from build123d import *

# Parameters (mm, degrees)
F0_W     = 254
F0_H     = 127
F1_DEPTH = 76.2
F2_W     = 25.4
F2_H     = 76.2
F3_DEPTH = 255.778
F5_D     = 38.1
F6_D     = 38.1
F7_D     = 38.1


with BuildPart() as f1:
    # F0 (on Front) → F1 (new body)
    with BuildSketch(Plane.XZ):
        with Locations((-2.316557, -18.004625)):
            Rectangle(F0_W, F0_H)
    extrude(amount=F1_DEPTH)

    # F2 (on face) → F3 (cut)
    with BuildSketch(Plane.YZ.offset(124.683443)):
        with Locations((-63.5, 7.395375)):
            Rectangle(F2_W, F2_H)
    extrude(amount=-F3_DEPTH, mode=Mode.SUBTRACT)

    # F5 (through all)
    with Locations(Plane.XZ.offset(50.8)):
        with Locations((-103.916557, 20.095375)):
            Hole(F5_D / 2)

    # F6 (through all)
    with Locations(Plane.XZ.offset(50.8)):
        with Locations((-53.116557, 20.095375)):
            Hole(F6_D / 2)

    # F7 (through all)
    with Locations(Plane.XZ.offset(50.8)):
        with Locations((-2.316557, 20.095375), (48.483443, 20.095375), (99.283443, 20.095375)):
            Hole(F7_D / 2)


solid = f1.part
Read the model definition and answer for the solid it produces. Units are mm, in the model's axes. A direction names the side the tool comes from. Coordinates: 2 decimals unless noted, no trailing zeros. Loops run counter-clockwise (first coordinate to the right, second up) from the corner with the lowest first, then second, coordinate; pieces in that order, holes last. Notation, with made-up numbers: (-27.75, -5) - (17.25, -5) arc R18 ccw to (17.25, -1) - close; hole circle Ø9 at (66.5, -29.75). An arc over 180 degrees is marked (long way). Answer in a Markdown table with one row per item.
Q1. Find section D-D on x = 100.5. Write down the section's boundary in (y, z).
Here are the results:
| item | result |
|---|---|
| outline | (-76.2, -81.5) - (0, -81.5) - (0, 1.08) - (-50.8, 1.08) - (-50.8, -30.7) - (-76.2, -30.7) - close; (-50.8, 39.11) - (0, 39.11) - (0, 45.5) - (-50.8, 45.5) - close |
Q2. Find section A-A on z = 31. Write down the section's boundary in (x, y), plus the area to 3 significant figures.
Here are the results:
| item | result |
|---|---|
| outline | (-129.32, -50.8) - (-119.54, -50.8) - (-119.54, 0) - (-129.32, 0) - close; (-88.3, -50.8) - (-68.74, -50.8) - (-68.74, 0) - (-88.3, 0) - close; (-37.5, -50.8) - (-17.94, -50.8) - (-17.94, 0) - (-37.5, 0) - close; (13.3, -50.8) - (32.86, -50.8) - (32.86, 0) - (13.3, 0) - close; (64.1, -50.8) - (83.66, -50.8) - (83.66, 0) - (64.1, 0) - close; (114.9, -50.8) - (124.68, -50.8) - (124.68, 0) - (114.9, 0) - close |
| area | 4,970 mm^2 |
Q3. For faces 4 (the flat face through (124.683, -29, -19)), 5 (the flat face through (-1, -50.8, -2)), determine the directions among +Z, -Z, +X, -X, +Y, -Y from which every point of the face is accessible in a straight line to the end or side of a thin tool.
Here are the results:
| item | result |
|---|---|
| face 4 | +Z, -Z, +X, +Y, -Y |
| face 5 | +Z, +X, -X, -Y |
Q4. The mould has two halves that part along Z. Classify faces 1 (the flat face through (-4, -76.2, -56)), 2 (the cylindrical face through (30.886, -25.044, 12.799)), 3 (the flat face through (-1, -64, -30.705)): pulls with the +Z half, pulls with the -Z half, needs draft (parallel to the pull), parting line crosses it, or undercut.
Here are the results:
| item | result |
|---|---|
| face 1 | needs draft |
| face 2 | undercut |
| face 3 | pulls with the +Z half |
Q5. Find section B-B on x = -15.5. Write down the section's boundary in (y, z), plus the area to 3 significant figures.
Here are the results:
| item | result |
|---|---|
| outline | (-76.2, -81.5) - (0, -81.5) - (0, 6.34) - (-50.8, 6.34) - (-50.8, -30.7) - (-76.2, -30.7) - close; (-50.8, 33.85) - (0, 33.85) - (0, 45.5) - (-50.8, 45.5) - close |
| area | 6,340 mm^2 |
Q6. Given P1, Ø23, axis at x = -23, z = 6.5, coming from the -Y side, flat-ended and moving along its own axis, determine where the tip first touches the part or whether it passes through.
Here are the results:
| item | result |
|---|---|
| P1 | stops at y = -50.8 |
Q7. Find section C-C on y = -13. Write down the section's boundary in (x, z), plus the area to 3 significant figures.
Here are the results:
| item | result |
|---|---|
| outline | (-129.32, -81.5) - (124.68, -81.5) - (124.68, 45.5) - (-129.32, 45.5) - close; hole circle Ø38.1 at (-103.92, 20.1); hole circle Ø38.1 at (-53.12, 20.1); hole circle Ø38.1 at (-2.32, 20.1); hole circle Ø38.1 at (48.48, 20.1); hole circle Ø38.1 at (99.28, 20.1) |
| area | 26,600 mm^2 |
Q8. Straight lines are drawn through the part: line 1 along X through (y, z) = (-46, 34.5); line 2 along Z through (x, y) = (-16, -47.5); line 3 along Y through (x, z) = (56, -10). For each, find the intervals that lie inside material, in ascending order. Write a range as [from, to].
Here are the results:
| item | result |
|---|---|
| line 1 | x = [-129.32, -116.38], [-91.45, -65.58], [-40.65, -14.78], [10.15, 36.02], [60.95, 86.82], [111.75, 124.68] |
| line 2 | z = [-81.5, 6.84], [33.35, 45.5] |
| line 3 | y = [-50.8, 0] |
